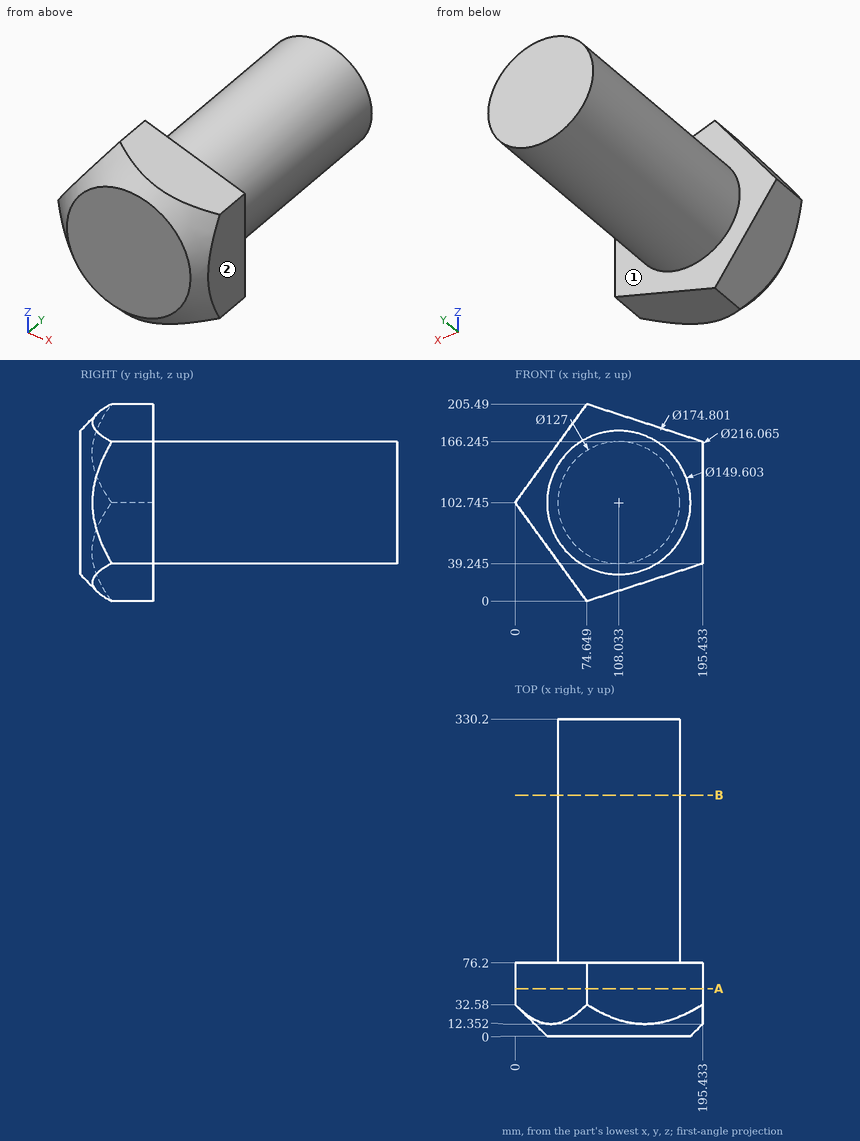
Input: dimensioned drawing with shaded views. Units: mm. Origin: part minimum x, y, z. A direction names the side the tool comes from. Give positions to 0.01 mm unless a question says otherwise; leave off trailing zeros. Loops run counter-clockwise (first coordinate to the right, second up) from the corner with the lowest first, then second, coordinate; pieces in that order, holes last. Notation, with made-up numbers: (29.25, 48) - (67.25, 48) arc R8 ccw to (67.25, 61) - close; hole circle Ø3 at (71, 88). An arc over 180 degrees is marked (long way). Answer as CSV lines item,"result". Start each with the question number.
(1) Section query B-B (y = 251). Output: boundary loops of the cut face in (x, z) (1 decimal).
(2) Ray query, line 1 along Y through (x, z) = (88, 171); line 2 along Z through (x, y) = (182.5, 35); line 3 along Z through (x, y) = (168.5, 63.5) (1 decimal). Return the intervals inside material, ascending. Write a range as [from, to].
(3) Reachability of the marked faces 1 and 2 from +Z, -Z, +X, -X, +Y, -Y: full face, straight path, thin tool, end or side. Return the list, or none.
(4) Pin query (flat end, axial travel): P1, Ø4, axis at x = 131.5, y = 276.5, coming from the -Z side (1 decimal); P2, Ø2, axis at x = 43.5, z = 43.5, coming from the -Y side; P3, Ø12, axis at x = 49.5, z = 177.5, coming from the -Y side (1 decimal). Return the tip coordinate at first contact, or that it passes through.
(5) Section query A-A (y = 49.5). Output: boundary loops of the cut face in (x, z) (1 decimal).
Worked answers:
1,outline,"circle Ø127 at (108, 102.7)"
2,line 1,"y = [0, 76.2]"
2,line 2,"z = [35.04, 170.45]"
2,line 3,"z = [30.5, 175]"
3,face 1,"+Y"
3,face 2,"+Z, -Z, +X, +Y, -Y"
4,P1,"stops at z = 43"
4,P2,"stops at y = 11.57"
4,P3,"stops at y = 13.9"
5,outline,"(0, 102.7) - (74.6, 0) - (195.4, 39.2) - (195.4, 166.2) - (74.6, 205.5) - close"
